Could you check a few things on this model? Use its own coordinates, in mm. Give positions to 0.01 mm unless a question says otherwise; leave off trailing zeros. Loops run counter-clockwise (first coordinate to the right, second up) from the corner with the lowest first, then second, coordinate; pieces in that order, holes last. Notation, with made-up numbers: (42, 3) - (98, 3) arc R28 ccw to (98, 23) - close; hole circle Ø3 at (64, 62). An arc over 180 degrees is marked (long way). Write each question's results on one line, items separated by ' | '. Start each with the question number.
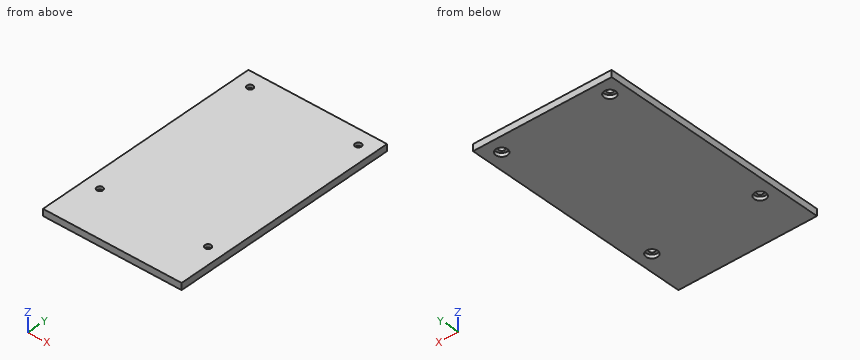
```python
from build123d import *

# Parameters (mm, degrees)
CYLINDER007_R     = 2.8
CYLINDER007_DEPTH = 1.75
CYLINDER006_R     = 2.8
CYLINDER006_DEPTH = 1.75
CYLINDER005_R     = 2.8
CYLINDER005_DEPTH = 1.75
CYLINDER004_R     = 2.8
CYLINDER004_DEPTH = 1.75
CYLINDER003_R     = 1.5
CYLINDER003_DEPTH = 10
CYLINDER002_R     = 1.5
CYLINDER002_DEPTH = 10
CYLINDER001_R     = 1.5
CYLINDER001_DEPTH = 10
CYLINDER_R        = 1.5
CYLINDER_DEPTH    = 10
BOX001_W          = 66.69
BOX001_H          = 111.14
BOX001_DEPTH      = 3.25


with BuildPart() as cylinder007:
    # Cylinder007 → Cylinder007 (new body)
    with BuildSketch(Plane(origin=(55.88, 100.33, 0), x_dir=(1, 0, 0), z_dir=(0, 0, 1))):
        Circle(CYLINDER007_R)
    extrude(amount=CYLINDER007_DEPTH)


with BuildPart() as cylinder006:
    # Cylinder006 → Cylinder006 (new body)
    with BuildSketch(Plane(origin=(3.81, 100.33, 0), x_dir=(1, 0, 0), z_dir=(0, 0, 1))):
        Circle(CYLINDER006_R)
    extrude(amount=CYLINDER006_DEPTH)


with BuildPart() as cylinder005:
    # Cylinder005 → Cylinder005 (new body)
    with BuildSketch(Plane(origin=(55.88, 19.05, 0), x_dir=(1, 0, 0), z_dir=(0, 0, 1))):
        Circle(CYLINDER005_R)
    extrude(amount=CYLINDER005_DEPTH)


with BuildPart() as cylinder004:
    # Cylinder004 → Cylinder004 (new body)
    with BuildSketch(Plane(origin=(3.81, 19.05, 0), x_dir=(1, 0, 0), z_dir=(0, 0, 1))):
        Circle(CYLINDER004_R)
    extrude(amount=CYLINDER004_DEPTH)


with BuildPart() as cylinder003:
    # Cylinder003 → Cylinder003 (new body)
    with BuildSketch(Plane(origin=(55.88, 100.33, -1), x_dir=(1, 0, 0), z_dir=(0, 0, 1))):
        Circle(CYLINDER003_R)
    extrude(amount=CYLINDER003_DEPTH)


with BuildPart() as cylinder002:
    # Cylinder002 → Cylinder002 (new body)
    with BuildSketch(Plane(origin=(3.81, 100.33, -1), x_dir=(1, 0, 0), z_dir=(0, 0, 1))):
        Circle(CYLINDER002_R)
    extrude(amount=CYLINDER002_DEPTH)


with BuildPart() as cylinder001:
    # Cylinder001 → Cylinder001 (new body)
    with BuildSketch(Plane(origin=(55.88, 19.05, -1), x_dir=(1, 0, 0), z_dir=(0, 0, 1))):
        Circle(CYLINDER001_R)
    extrude(amount=CYLINDER001_DEPTH)


with BuildPart() as cylinder:
    # Cylinder → Cylinder (new body)
    with BuildSketch(Plane(origin=(3.81, 19.05, -1), x_dir=(1, 0, 0), z_dir=(0, 0, 1))):
        Circle(CYLINDER_R)
    extrude(amount=CYLINDER_DEPTH)


with BuildPart() as cut007:
    # Box001 → Box001 (new body)
    with BuildSketch(Plane(origin=(-3.5, -3.5, 0), x_dir=(1, 0, 0), z_dir=(0, 0, 1))):
        with Locations((33.345, 55.57)):
            Rectangle(BOX001_W, BOX001_H)
    extrude(amount=BOX001_DEPTH)

    # Cut: cut Cylinder
    add(cylinder.part, mode=Mode.SUBTRACT)

    # Cut001: cut Cylinder001
    add(cylinder001.part, mode=Mode.SUBTRACT)

    # Cut002: cut Cylinder002
    add(cylinder002.part, mode=Mode.SUBTRACT)

    # Cut003: cut Cylinder003
    add(cylinder003.part, mode=Mode.SUBTRACT)

    # Cut004: cut Cylinder004
    add(cylinder004.part, mode=Mode.SUBTRACT)

    # Cut005: cut Cylinder005
    add(cylinder005.part, mode=Mode.SUBTRACT)

    # Cut006: cut Cylinder006
    add(cylinder006.part, mode=Mode.SUBTRACT)

    # Cut007: cut Cylinder007
    add(cylinder007.part, mode=Mode.SUBTRACT)


solid = cut007.part
```
Q1. I want a section at A-A, the plane y = 19.05. List the corners of the cut face in (x, z) for me.
Q2. I need wall thicknesses on L1, parallel to Y at x = 3.81, z = 2.95; L2, parallel to Y at x = 3.81, z = 1.05; L3, parallel to X at y = 19.05, z = 2.55. Which ranges of each line are inside material? Lowest first, please. Write a range as from..to.
Q3. I want a section at B-B, the plane x = 55.88. List the corners of the cut face in (y, z) for me, then the cut area to 3 significant figures.
Q4. I'm going to push flat-ended pins straight in: pin 1 Ø5 at (x, y) = (3.81, 19.05) entering from -Z; pin 2 Ø2.5 at (x, y) = (55.88, 100.33) entering from +Z. Where does each tip first touch, or does it pass through?
Conclusion:
1) outline: (-3.5, 0) - (1.01, 0) - (1.01, 1.75) - (2.31, 1.75) - (2.31, 3.25) - (-3.5, 3.25) - close; (5.31, 1.75) - (6.61, 1.75) - (6.61, 0) - (53.08, 0) - (53.08, 1.75) - (54.38, 1.75) - (54.38, 3.25) - (5.31, 3.25) - close; (57.38, 1.75) - (58.68, 1.75) - (58.68, 0) - (63.19, 0) - (63.19, 3.25) - (57.38, 3.25) - close
2) L1: -3.5..17.55, 20.55..98.83, 101.83..107.64 | L2: -3.5..16.25, 21.85..97.53, 103.13..107.64 | L3: -3.5..2.31, 5.31..54.38, 57.38..63.19
3) outline: (-3.5, 0) - (16.25, 0) - (16.25, 1.75) - (17.55, 1.75) - (17.55, 3.25) - (-3.5, 3.25) - close; (20.55, 1.75) - (21.85, 1.75) - (21.85, 0) - (97.53, 0) - (97.53, 1.75) - (98.83, 1.75) - (98.83, 3.25) - (20.55, 3.25) - close; (101.83, 1.75) - (103.13, 1.75) - (103.13, 0) - (107.64, 0) - (107.64, 3.25) - (101.83, 3.25) - close | area: 333 mm^2
4) pin 1: z = 1.75 | pin 2: through
